The listing builds one solid part. Answer for the finished solid, in the listing's coordinates (mm). Coordinates: 2 decimals unless noted, no trailing zeros. Order: outer loops, then holes, each group sorted by start corner. A loop starts at its lowest first (then second) coordinate and runs counter-clockwise, first axis right, second up. Notation, with made-up numbers: (72.5, -13) - (100.5, -13) arc R21 ccw to (100.5, -1) - close; hole circle Ø1 at (51, 67.25). An arc over 180 degrees is marked (long way). Use one line per item in the form item = value. Start each with the question number.
Item 1: Section C-C, the plane z = 0.9 is taken. Count the separate pieces of the cut face and the enclosed holes in it, and give its area (3 significant figures).
Item 2: Section D-D, the plane y = -64 is taken. Write down the section's boundary in (x, z), and give its area (4 significant figures).
Item 3: Section A-A, the plane x = 20 is taken. Write down the section's boundary in (y, z), and give its area (3 significant figures).
Item 4: Each of these flat-tipped pins is pushed along its axis until it touches: pin 1 Ø1.5 at (x, z) = (56.5, 1) entering from +Y; pin 2 Ø0.9 at (y, z) = (-23, 2) entering from +X; pin 3 Ø1.5 at (y, z) = (1.5, 1) entering from -X; pin 4 Ø1.5 at (x, y) = (43.5, -5) entering from +Z. Where does it stop, or does it pass through?
Item 5: Consider line 1 along Y through (x, z) = (43.5, 1.9); line 2 along X through (y, z) = (-31, 0.5); line 3 along Y through (x, z) = (2, 1.9). Determine where each line is inside the solid, lowest interval first. Write a range as [from, to].
Item 6: Section B-B, the plane y = -10 is taken. Write down the section's boundary in (x, z), and give its area (3 significant figures).
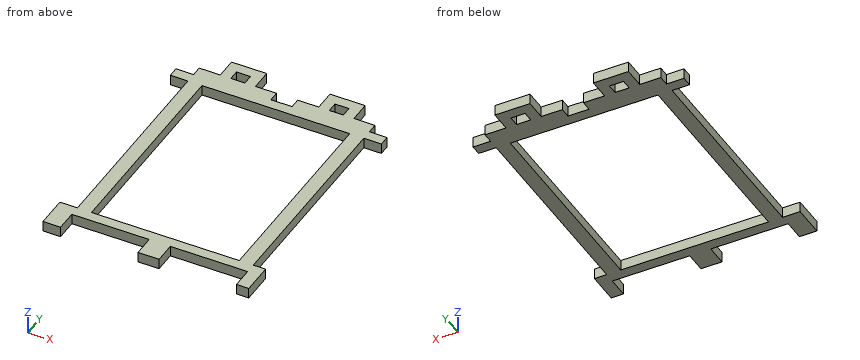
from build123d import *

# Parameters (mm, degrees)
SKETCH1_W           = 42
SKETCH1_H           = 59
BOSS_EXTRUDE1_DEPTH = 3
BOSS_EXTRUDE2_DEPTH = 3


with BuildPart() as part:
    # Sketch1 → Boss-Extrude1 (new body)
    with BuildSketch(Plane.XY):
        Polygon((0, 0), (5, 0), (5, 3), (27, 3), (27, 0), (33, 0), (33, 3), (55, 3), (55, 0), (60, 0), (60, -3), (55, -3), (55, -62), (58.5, -62), (58.5, -71), (55, -71), (55, -65), (33, -65), (33, -71), (27, -71), (27, -65), (5, -65), (5, -71), (0, -71), (0, -62), (5, -62), (5, -3), (0, -3), align=None)
        with Locations((30, -32.5)):
            Rectangle(SKETCH1_W, SKETCH1_H, mode=Mode.SUBTRACT)
    extrude(amount=BOSS_EXTRUDE1_DEPTH)

    # Sketch2 → Boss-Extrude2 (add)
    with BuildSketch(Plane(origin=(0, 0, 0), x_dir=(-1, 0, 0), z_dir=(0, 0, -1))):
        Polygon((-49, 9), (-49, 3), (-46, 3), (-46, 6), (-42, 6), (-42, 3), (-39, 3), (-39, 9), align=None)
        Polygon((-21, 3), (-18, 3), (-18, 6), (-14, 6), (-14, 3), (-11, 3), (-11, 9), (-21, 9), align=None)
    extrude(amount=-BOSS_EXTRUDE2_DEPTH)


solid = part.part
Response:
q1.separate_pieces = 1
q1.enclosed_holes = 3
q1.area = 1,140 mm2
q2.outline = (0, 0) - (58.5, 0) - (58.5, 3) - (0, 3) - close
q2.area = 175.5 mm2
q3.outline = (-65, 0) - (-62, 0) - (-62, 3) - (-65, 3) - close; (-3, 0) - (9, 0) - (9, 3) - (-3, 3) - close
q3.area = 45.0 mm2
q4.pin_1 = 0
q4.pin_2 = 55
q4.pin_3 = 5
q4.pin_4 = through
q5.line_1 = [-65, -62], [-3, 3], [6, 9]
q5.line_2 = [5, 9], [51, 55]
q5.line_3 = [-71, -62], [-3, 0]
q6.outline = (5, 0) - (9, 0) - (9, 3) - (5, 3) - close; (51, 0) - (55, 0) - (55, 3) - (51, 3) - close
q6.area = 24.0 mm2
